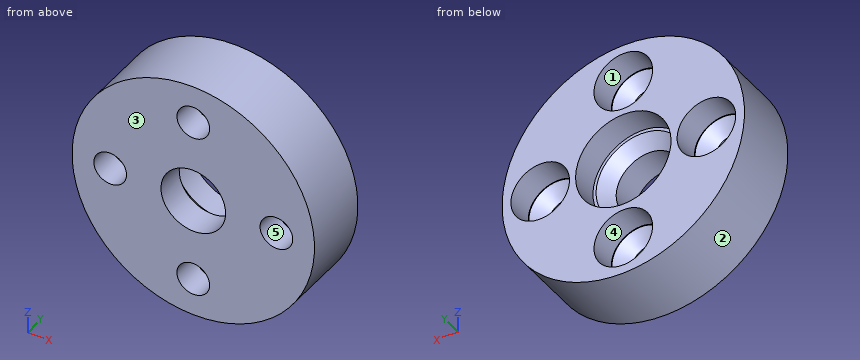
from build123d import *

# Parameters (mm, degrees)
SKETCH1_R           = 8.89
SKETCH1_R_2         = 2.37125
SKETCH1_R_3         = 1.2
BOSS_EXTRUDE1_DEPTH = 5
SKETCH2_R           = 2.15
SKETCH2_R_2         = 3.5
CUT_EXTRUDE1_DEPTH  = 2
CHAMFER1_SIZE       = 0.9


with BuildPart() as part:
    # Sketch1 → Boss-Extrude1 (new body)
    with BuildSketch(Plane(origin=(0, 0, 0), x_dir=(1, 0, 0), z_dir=(0, 1, 0))):
        with Locations(Location((0, 0, 0), (0, 0, 270))):
            Circle(SKETCH1_R)
        with Locations(Location((0, 0, 0), (0, 0, 270))):
            Circle(SKETCH1_R_2, mode=Mode.SUBTRACT)
        with Locations(Location((0, -6.096, 0), (0, 0, 270))):
            Circle(SKETCH1_R_3, mode=Mode.SUBTRACT)
        with Locations(Location((-6.096, 0, 0), (0, 0, 270))):
            Circle(SKETCH1_R_3, mode=Mode.SUBTRACT)
        with Locations(Location((0, 6.096, 0), (0, 0, 270))):
            Circle(SKETCH1_R_3, mode=Mode.SUBTRACT)
        with Locations(Location((6.096, 0, 0), (0, 0, 270))):
            Circle(SKETCH1_R_3, mode=Mode.SUBTRACT)
    extrude(amount=BOSS_EXTRUDE1_DEPTH)

    # Sketch2 → Cut-Extrude1 (cut)
    with BuildSketch(Plane(origin=(0, 5, 0), x_dir=(1, 0, 0), z_dir=(0, 1, 0))):
        with Locations(Location((0, 6.096, 0), (0, 0, 270))):
            Circle(SKETCH2_R)
        with Locations(Location((-6.096, 0, 0), (0, 0, 270))):
            Circle(SKETCH2_R)
        with Locations(Location((6.096, 0, 0), (0, 0, 270))):
            Circle(SKETCH2_R)
        with Locations(Location((0, -6.096, 0), (0, 0, 270))):
            Circle(SKETCH2_R)
        with Locations(Location((0, 0, 0), (0, 0, 270))):
            Circle(SKETCH2_R_2)
    extrude(amount=-CUT_EXTRUDE1_DEPTH, mode=Mode.SUBTRACT)

    # Chamfer1
    chamfer1_edges = [part.edges().sort_by_distance(p)[0] for p in [
        (0, 3, -7.296),
        (0, 3, -2.37125),
        (0, 3, 4.896),
        (6.096, 3, -1.2),
        (-6.096, 3, -1.2),
    ]]
    chamfer(chamfer1_edges, length=CHAMFER1_SIZE)


solid = part.part
Input: part model. Units: mm. Frame: model coordinates. Face numbers are marked on the shaded views. A direction names the side the tool comes from. Coordinates: 2 decimals unless noted, no trailing zeros. Order: outer loops, then holes, each group sorted by start corner. A loop starts at its lowest first (then second) coordinate and runs counter-clockwise, first axis right, second up. Notation, with made-up numbers: M -39,-22 L 13,-22 A12 ccw 13,-11 Z; hole C 29.5,-0.5 d6. An arc over 180 degrees is marked long. Answer in a Markdown table with one row per item.
(1) Section query A-A, the plane z = 0. Give the number of separate pieces and of enclosed holes in the cut face, plus the area to 3 significant figures.
Numbers:
| item | result |
|---|---|
| separate pieces | 4 |
| enclosed holes | 0 |
| area | 26.6 mm^2 |
(2) Access query for the marked faces 4 and 5. Directions: +Z, -Z, +X, -X, +Y, -Y. A direction counts if a zero-diameter tool reaches every point of the face in a straight line with its end or side. Return the directions, or none.
Numbers:
| item | result |
|---|---|
| face 4 | +Y |
| face 5 | +Y, -Y |
(3) Draft query along Z for the marked faces 1, 2 and 3. Return one class per face: pulls with the +Z half, pulls with the -Z half, needs draft (parallel to the pull), parting line crosses it, or undercut.
Numbers:
| item | result |
|---|---|
| face 1 | undercut |
| face 2 | parting line crosses it |
| face 3 | needs draft |
(4) Contact query for flat-ended pins moving along their axis: pin 1 Ø3.5 at (x, z) = (-6.5, 0.5) entering from +Y; pin 2 Ø4 at (x, z) = (0, -6.096) entering from +Y; pin 3 Ø2 at (x, y) = (-7, 2.5) entering from +Z; pin 4 Ø1.3 at (x, z) = (6, 1) entering from +Y. Output: stop coordinate, or through.
Numbers:
| item | result |
|---|---|
| pin 1 | stops at y = 5 |
| pin 2 | stops at y = 2.9 |
| pin 3 | stops at z = 6.56 |
| pin 4 | stops at y = 2.55 |
(5) Material intervals for line 1 (X direction, y = 4.2, z = 0); line 2 (X direction, y = 1.7, z = 0); line 3 (Z direction, x = 1, y = 2.55), sorted ascending. Write a range as [from, to].
Numbers:
| item | result |
|---|---|
| line 1 | x = [-8.89, -8.25], [-3.95, -3.5], [3.5, 3.95], [8.25, 8.89] |
| line 2 | x = [-8.89, -7.3], [-4.9, -2.37], [2.37, 4.9], [7.3, 8.89] |
| line 3 | z = [-8.83, -7.41], [-4.78, -2.64], [2.64, 4.78], [7.41, 8.83] |
(6) Section query C-C, the plane y = 1.7. Output: boundary loops of the cut face in (x, z).
Numbers:
| item | result |
|---|---|
| outline | C 0,0 d17.78; hole C -6.1,0 d2.4; hole C 0,0 d4.74; hole C 0,-6.1 d2.4; hole C 0,6.1 d2.4; hole C 6.1,0 d2.4 |
